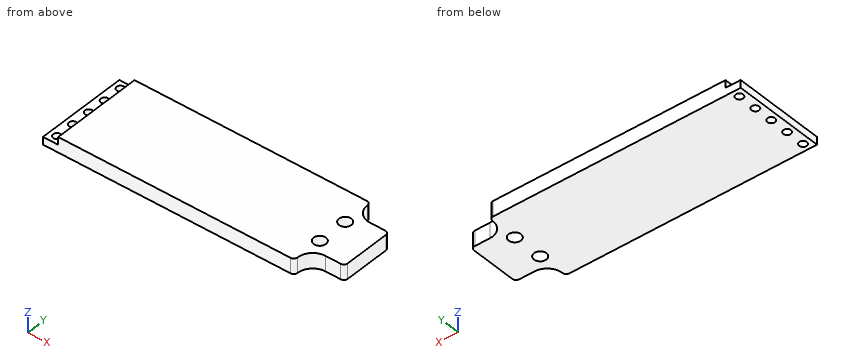
Autodesk Inventor part; units mm, degrees
ref_plane "YZ Plane" through (0, 0, 0) normal (1, 0, 0) x (0, 1, 0)
ref_plane "XZ Plane" through (0, 0, 0) normal (0, 1, 0) x (-1, 0, 0)
ref_plane "XY Plane" through (0, 0, 0) normal (0, 0, 1) x (1, 0, 0)
sketch "Skizze1" plane through (0, 0, 0) normal (0, 0, 1) x (1, 0, 0)
  line L0 (0, 12) -> (66, 12)
  line L1 (66, -12) -> (0, -12)
  line L2 (0, -12) -> (0, 12)
  line L3 (-15, 0) -> (90, 0)
  line L4 (66, -7) -> (75, -7)
  line L5 (75, -7) -> (75, 7)
  line L6 (75, 7) -> (66, 7)
  line L7 (66, 12) -> (66, 7)
  line L8 (66, -7) -> (66, -12)
  point P0 (0, 0)
  dimension "d0" = 24
  dimension "d1" = 66
  dimension "d29" = 14
  dimension "d30" = 9
extrude "Extrusion1" add sketch "Skizze1" along normal blind 4
sketch "Skizze2" plane through (0, 0, 4) normal (0, 0, 1) x (1, 0, 0)
  line L0 (66, 12) -> (0, 12)
  line L1 (0, 12) -> (0, -12)
  line L2 (0, 12) -> (4, 12)
  line L3 (4, 12) -> (4, -12)
  line L4 (4, -12) -> (0, -12)
  line L5 (0, -12) -> (0, 12)
  point P0 (0, 0)
  dimension "d4" = 4
extrude "Extrusion2" cut sketch "Skizze2" against normal blind 2
sketch "Skizze3" plane through (0, 0, 2) normal (0, 0, 1) x (1, 0, 0)
  line L0 (0, 16.8) -> (0, -16.8)
  line L1 (-15, 0) -> (90, 0)
  point P0 (0, 0)
  point P1 (2, 0)
  dimension "d7" = 2
hole "Bohrung1" at (2, 0, 2) direction (0, 0, -1) diameter 2 end through all
pattern_linear "Rechteckige Anordnung1" count 5 spacing 5 along (0, 1, 0) of "Bohrung1" first direction both ways yes
sketch "Skizze4" plane through (0, 0, 4) normal (0, 0, 1) x (1, 0, 0)
  line L0 (-15, 0) -> (90, 0)
  line L1 (66, -12) -> (66, 12)
  line L2 (75, -7) -> (75, 7) construction
  point P0 (0, 0)
  point P1 (66, 4)
  point P2 (66, -4)
  dimension "d31" = 8
  dimension "d36" = 0
hole "Bohrung2" at (66, -4, 4) at (66, 4, 4) direction (0, 0, -1) diameter 3.242 end through all
fillet "Rundung1" radius 4 2 edges at (66, -7, 2) (66, 7, 2)
fillet "Rundung2" radius 1 4 edges at (66, -12, 2) (66, 12, 2) (75, -7, 2) (75, 7, 2)
properties part number "Kicker Eisen" material "Stahl, unlegiert"
Read the model definition and answer for the solid it produces. Units are mm, in the model's axes. Give positions to 0.01 mm unless a question says otherwise; leave off trailing zeros. Write each loop counter-clockwise with the first axis right and the second up, starting at its lowest first coordinate (ties: lowest second). Pieces come first, ordered by that corner, then holes. Notation, with made-up numbers: M 51,21 L 64,21 A26 cw 64,49 Z; hole C 45,-38 d2. An arc over 180 degrees is marked long. One line per item, written item: value. Start each with the question number.
(1) Find section B-B (y = 0). Determine the outline of the cut face in (x, z), plus the area to 3 significant figures.
(2) Flat-ended cylindrical pins translate along their axes: pin 1 Ø1.2 at (x, z) = (71.5, 1) entering from +Y; pin 2 Ø2 at (y, z) = (4.5, 3.5) entering from -X; pin 3 Ø1.2 at (x, z) = (73, 1.5) entering from -Y. Find the tip coordinate at first contact, or state that the pin passes through.
(3) Find the intervals of material crossed by line 1 (Y direction, x = 65, z = 3.85); line 2 (Y direction, x = 2, z = 0.45); line 3 (X direction, y = 5, z = 0.6), in increasing order.
(4) Find section A-A (x = 2). Determine the outline of the cut face in (y, z), plus the area to 3 significant figures.
(5) Find section D-D (y = -10). Determine the outline of the cut face in (x, z).
(6) Find section C-C (z = 1.1). Give the number of separate pieces and of enclosed holes in the cut face, plus the area to 3 significant figures.
Results below:
1. outline: M 0,0 L 1,0 L 1,2 L 0,2 Z; M 3,0 L 75,0 L 75,4 L 4,4 L 4,2 L 3,2 Z
1. area: 288 mm^2
2. pin 1: stops at y = 7
2. pin 2: stops at x = 4
2. pin 3: stops at y = -7
3. line 1: y = -12 to -5.28, -2.72 to 2.72, 5.28 to 12
3. line 2: y = -12 to -11, -9 to -6, -4 to -1, 1 to 4, 6 to 9, 11 to 12
3. line 3: x = 0 to 1, 3 to 64.72, 67.28 to 75
4. outline: M -12,0 L -11,0 L -11,2 L -12,2 Z; M -9,0 L -6,0 L -6,2 L -9,2 Z; M -4,0 L -1,0 L -1,2 L -4,2 Z; M 1,0 L 4,0 L 4,2 L 1,2 Z; M 6,0 L 9,0 L 9,2 L 6,2 Z; M 11,0 L 12,0 L 12,2 L 11,2 Z
4. area: 28.0 mm^2
5. outline: M 0,0 L 1,0 L 1,2 L 0,2 Z; M 3,0 L 66.13,0 L 66.13,4 L 4,4 L 4,2 L 3,2 Z
6. separate pieces: 1
6. enclosed holes: 7
6. area: 1,680 mm^2
